from build123d import *

# Parameters (mm, degrees)
CUT_EXTRUDE3_DEPTH           = 60
CUT_EXTRUDE5_DEPTH           = 2
CUT_EXTRUDE5_DEPTH_BACK      = 30
SKETCH9_R                    = 38
SKETCH9_R_2                  = 23
SKETCH19_W                   = 12
SKETCH19_H                   = 36.5
CUT_REVOLVE2_ANGLE           = 65
CUT_REVOLVE2_OTHER_WAY_ANGLE = 65
SKETCH21_W                   = 3.25
SKETCH21_H                   = 4
BOSS_EXTRUDE3_DEPTH          = 1.35
CIRPATTERN1_COUNT            = 5
CUT_EXTRUDE9_START           = -5
CUT_EXTRUDE9_DEPTH           = 5
SKETCH23_R                   = 10.5
CUT_EXTRUDE10_DEPTH          = 10
SKETCH24_W                   = 15
SKETCH24_H                   = 8
BOSS_EXTRUDE4_DEPTH          = 8
SKETCH26_W                   = 10
SKETCH26_H                   = 6
CUT_EXTRUDE11_DEPTH          = 10
SKETCH27_W                   = 4
SKETCH27_H                   = 5
CUT_EXTRUDE12_DEPTH          = 5
CUT_EXTRUDE14_DEPTH          = 2
CUT_EXTRUDE14_DEPTH_BACK     = 30
SKETCH29_R                   = 1
CUT_EXTRUDE15_DEPTH          = 15
FILLET1_R                    = 6
FILLET2_R                    = 8
INTERSECT1_DEPTH             = 58.427876097
SKETCH31_W                   = 6
SKETCH31_H                   = 3
BOSS_EXTRUDE7_DEPTH          = 8


# Read off the part's stored shape, not the designer's step: Cut-Extrude9, Intersect1
with BuildPart() as part:
    # Sketch1 → Revolve1 (revolve)
    with BuildSketch(Plane.XY, mode=Mode.PRIVATE) as revolve1_sk:
        with BuildLine():
            Line((0, 63.427876097), (32, 63.427876097))
            ThreePointArc((32, 63.427876097), (37.656854249, 61.084730346), (40, 55.427876097))
            Line((40, 55.427876097), (40, 28.846818009))
            ThreePointArc((40, 28.846818009), (38.792081772, 24.082439968), (35.460140376, 20.469057744))
            Line((35.460140376, 20.469057744), (28.539859624, 15.958818353))
            ThreePointArc((28.539859624, 15.958818353), (25.207918228, 12.345436129), (24, 7.581058088))
            Line((24, 7.581058088), (24, 3.25))
            Line((24, 3.25), (24.35, 3))
            Line((24.35, 3), (24.35, 0))
            Line((24.35, 0), (22.5, 0))
            Line((22.5, 0), (22.5, 12.5))
            ThreePointArc((22.5, 12.5), (22.353553391, 12.853553391), (22, 13))
            Line((22, 13), (0, 13))
            Line((0, 13), (0, 63.427876097))
        make_face()
    revolve(revolve1_sk.sketch.rotate(Axis((0, 0, 0), (0, 1, 0)), 90), axis=Axis((0, 0, 0), (0, 1, 0)))

    # Sketch11 → Cut-Extrude3 (cut)
    with BuildSketch(Plane(origin=(0, 13, 0), x_dir=(-1, 0, 0), z_dir=(0, -1, 0))):
        with BuildLine():
            Line((-21, 0), (21, 0))
            ThreePointArc((21, 0), (0, 21), (-21, 0))
        make_face()
    extrude(amount=-CUT_EXTRUDE3_DEPTH, mode=Mode.SUBTRACT)

    # Sketch9 → Cut-Extrude5 (cut, two sides: drawn at the far end of the back side and taken through both)
    with BuildSketch(Plane(origin=(0, 55.427876097, 0), x_dir=(1, 0, 0), z_dir=(0, 1, 0)).offset(-CUT_EXTRUDE5_DEPTH_BACK)):
        with Locations(Location((0, 0, 0), (0, 0, 270))):
            Circle(SKETCH9_R)
        with Locations(Location((0, 0, 0), (0, 0, 270))):
            Circle(SKETCH9_R_2, mode=Mode.SUBTRACT)
    extrude(amount=CUT_EXTRUDE5_DEPTH + CUT_EXTRUDE5_DEPTH_BACK, mode=Mode.SUBTRACT)

    # Sketch19 → Cut-Revolve2 (revolve, cut)
    with BuildSketch(Plane(origin=(0, 0, 0), x_dir=(0, 0, -1), z_dir=(1, 0, 0))):
        with Locations((-41.064715832, 37.177876097)):
            Rectangle(SKETCH19_W, SKETCH19_H)
    revolve(axis=Axis((0, 0, 0), (0, 1, 0)), revolution_arc=CUT_REVOLVE2_ANGLE, mode=Mode.SUBTRACT)

    # Sketch19 → Cut-Revolve2 other way (revolve, cut)
    with BuildSketch(Plane(origin=(0, 0, 0), x_dir=(0, 0, -1), z_dir=(1, 0, 0))):
        with Locations((-41.064715832, 37.177876097)):
            Rectangle(SKETCH19_W, SKETCH19_H)
    revolve(axis=Axis((0, 0, 0), (0, -1, 0)), revolution_arc=CUT_REVOLVE2_OTHER_WAY_ANGLE, mode=Mode.SUBTRACT)

    # Sketch21 → Boss-Extrude3 (add)
    with BuildSketch(Plane(origin=(0, 0, 22.5), x_dir=(-1, 0, 0), z_dir=(0, 0, -1))):
        with Locations((0, 2)):
            Rectangle(SKETCH21_W, SKETCH21_H)
    boss_extrude3 = extrude(amount=BOSS_EXTRUDE3_DEPTH)

    # CirPattern1: Boss-Extrude3 ×5 about axis
    cirpattern1_axis = Axis((0, 0, 0), (0, 1, 0))
    for i in range(1, CIRPATTERN1_COUNT):
        add(boss_extrude3.rotate(cirpattern1_axis, i * 360 / CIRPATTERN1_COUNT))

    # Cut-Extrude9 outline → Cut-Extrude9 (cut)
    with BuildSketch(Plane(origin=(0, 63.427876097, 0), x_dir=(1, 0, 0), z_dir=(0, 1, 0)).offset(CUT_EXTRUDE9_START)):
        with BuildLine():
            ThreePointArc((40, 0), (0, 40), (-40, 0))
            Line((-40, 0), (-21, 0))
            ThreePointArc((-21, 0), (0, 21), (21, 0))
            Line((21, 0), (40, 0))
        make_face()
    extrude(amount=CUT_EXTRUDE9_DEPTH, mode=Mode.SUBTRACT)

    # Sketch23 → Cut-Extrude10 (cut)
    with BuildSketch(Plane(origin=(0, 0, -40), x_dir=(-1, 0, 0), z_dir=(0, 0, -1))):
        with Locations((0, 42.137876097)):
            Circle(SKETCH23_R)
    extrude(amount=-CUT_EXTRUDE10_DEPTH, mode=Mode.SUBTRACT)

    # Sketch24 → Boss-Extrude4 (add)
    with BuildSketch(Plane(origin=(0, 58.427876097, 0), x_dir=(1, 0, 0), z_dir=(0, 1, 0))):
        with Locations((0, 30)):
            Rectangle(SKETCH24_W, SKETCH24_H)
    extrude(amount=-BOSS_EXTRUDE4_DEPTH)

    # Sketch26 → Cut-Extrude11 (cut)
    with BuildSketch(Plane(origin=(0, 58.427876097, 0), x_dir=(1, 0, 0), z_dir=(0, 1, 0))):
        with Locations((0, 30)):
            Rectangle(SKETCH26_W, SKETCH26_H)
    extrude(amount=-CUT_EXTRUDE11_DEPTH, mode=Mode.SUBTRACT)

    # Sketch27 → Cut-Extrude12 (cut)
    with BuildSketch(Plane(origin=(7.5, 0, 0), x_dir=(0, 0, -1), z_dir=(1, 0, 0))):
        with Locations((30, 53.927876097)):
            Rectangle(SKETCH27_W, SKETCH27_H)
    extrude(amount=-CUT_EXTRUDE12_DEPTH, mode=Mode.SUBTRACT)

    # Sketch28 → Cut-Extrude14 (cut, two sides: drawn at the far end of the back side and taken through both)
    with BuildSketch(Plane(origin=(0, 55.427876097, 0), x_dir=(1, 0, 0), z_dir=(0, 1, 0)).offset(-CUT_EXTRUDE14_DEPTH_BACK)):
        with BuildLine():
            Line((-22.912878475, -2), (22.912878475, -2))
            ThreePointArc((22.912878475, -2), (0, -23), (-22.912878475, -2))
        make_face()
    extrude(amount=CUT_EXTRUDE14_DEPTH + CUT_EXTRUDE14_DEPTH_BACK, mode=Mode.SUBTRACT)

    # Sketch29 → Cut-Extrude15 (cut)
    with BuildSketch(Plane(origin=(0, 0, 0), x_dir=(-1, 0, 0), z_dir=(0, 0, -1))):
        with Locations((-30.416198487, 60.927876097)):
            Circle(SKETCH29_R)
        with Locations((30.416198487, 60.927876097)):
            Circle(SKETCH29_R)
        with Locations((0, 60.927876097)):
            Circle(SKETCH29_R)
    extrude(amount=-CUT_EXTRUDE15_DEPTH, mode=Mode.SUBTRACT)

    # Fillet1
    fillet1_edges = [part.edges().sort_by_distance(p)[0] for p in [
        (21, 35.713938048, 0),
        (-21, 35.713938048, 0),
    ]]
    fillet(fillet1_edges, radius=FILLET1_R)

    # Fillet2
    fillet2_edges = [part.edges().sort_by_distance(p)[0] for p in [
        (-22.912878475, 41.427876097, 2),
        (22.912878475, 41.427876097, 2),
    ]]
    fillet(fillet2_edges, radius=FILLET2_R)

    # Intersect1 outline → Intersect1 (cut)
    with BuildSketch(Plane(origin=(0, 0, 0), x_dir=(1, 0, 0), z_dir=(0, 1, 0))):
        with BuildLine():
            Line((-37.508702776, -13.895942431), (-42, -15.355253362))
            Line((-42, -15.355253362), (-42, -41))
            Line((-42, -41), (42, -41))
            Line((42, -41), (42, -15.355253362))
            Line((42, -15.355253362), (37.508702776, -13.895942431))
            ThreePointArc((37.508702776, -13.895942431), (0, 40), (-37.508702776, -13.895942431))
        make_face()
        with BuildLine():
            ThreePointArc((19.246817919, 8.4), (18.767687244, 2.713664655), (13.747727085, 0))
            Line((13.747727085, 0), (-13.747727085, 0))
            ThreePointArc((-13.747727085, 0), (-18.767687244, 2.713664655), (-19.246817919, 8.4))
            ThreePointArc((-19.246817919, 8.4), (0, 21), (19.246817919, 8.4))
        make_face(mode=Mode.SUBTRACT)
    extrude(amount=INTERSECT1_DEPTH, mode=Mode.SUBTRACT)

    # Sketch31 → Boss-Extrude7 (add)
    with BuildSketch(Plane(origin=(0, 58.427876097, 0), x_dir=(1, 0, 0), z_dir=(0, 1, 0))):
        with Locations((0, -30)):
            Rectangle(SKETCH31_W, SKETCH31_H)
    extrude(amount=-BOSS_EXTRUDE7_DEPTH)


solid = part.part
Could you check a few things on this model? Use its own coordinates, in mm. A direction names the side the tool comes from. Round coordinates to 2 decimals unless told otherwise and drop trailing zeros. Write each loop counter-clockwise with the first axis right and the second up, starting at its lowest first coordinate (ties: lowest second). Pieces come first, ordered by that corner, then holes. Notation, with made-up numbers: (-24.75, 77) -> (28.25, 77) arc R23 cw to (28.25, 89) -> close; hole circle Ø11 at (1, 9). An arc over 180 degrees is marked (long way). Use a Markdown table: item, result.
1. If we section it at A-A (x = 0): List the corners of the cut face in (y, z) for me.
Answer key:
| item | result |
|---|---|
| outline | (50.43, 28.5) -> (58.43, 28.5) -> (58.43, 0) -> (59.93, 0) -> (59.93, 15) -> (61.93, 15) -> (61.93, 0) -> (63.43, 0) -> (63.43, 32) arc R8 ccw to (58.43, 39.42) -> (58.43, 31.5) -> (50.43, 31.5) -> close |
2. If we section it at B-B (y = 55.25): List the corners of the cut face in (x, z) for me, then the cut area to 3 significant figures.
Answer key:
| item | result |
|---|---|
| outline | (-3, 28.5) -> (3, 28.5) -> (3, 31.5) -> (-3, 31.5) -> close |
| area | 18.0 mm^2 |
3. We'd pull the mould along Y, two halves only. Please class faces 1 (the face through (-30.2, 59.95, 7.4)), 2 (the face through (0, 50.428, 30)), 3 (the face through (0, 54, 28.5)): +Y half, -Y half, draft (parallel to the pull), parting line (faces both ways), or undercut.
Answer key:
| item | result |
|---|---|
| face 1 | undercut |
| face 2 | -Y half |
| face 3 | draft |
4. Please list where these lines run through material, in increasing order: probe 1 along Y at (x, z) = (0, 5.75); probe 2 along X at (y, z) = (60.5, 10); probe 3 along Y at (x, z) = (8.5, 18).
Answer key:
| item | result |
|---|---|
| probe 1 | y = 58.43 to 59.93, 61.93 to 63.43 |
| probe 2 | x = -36.85 to -31.32, -29.51 to -0.9, 0.9 to 29.51, 31.32 to 36.85 |
| probe 3 | y = 58.43 to 63.43 |
5. Which directions (+Z, -Z, +X, -X, +Y, -Y) give clear straight access to the entire face, cutting with the end or side of a thin tool? Please do faces 4 (the face through (0, 54, 31.5)), 5 (the face through (3, 54, 30)), 6 (the face through (0.217, 59.952, 7.395)).
Answer key:
| item | result |
|---|---|
| face 4 | +Z, +X, -X, -Y |
| face 5 | +Z, -Z, +X, -Y |
| face 6 | -Z |
6. For pin 1 Ø2 at (x, y) = (30, 61) entering from -Z; pin 2 Ø5 at (x, z) = (22, 19) entering from -Y; pin 3 Ø1.2 at (x, y) = (0, 60.93) entering from +Z; pin 4 Ø1 at (x, y) = (0, 61) entering from -Z, each with a flat end and sliding along its axis, tell me the tip position at first contact or that it passes through.
Answer key:
| item | result |
|---|---|
| pin 1 | stops at z = 0 |
| pin 2 | stops at y = 58.43 |
| pin 3 | stops at z = 38.32 |
| pin 4 | stops at z = 15 |
